Check sheet for the modelled part. Datum: model origin and axes. Units: mm. Face numbers are marked on the shaded views. A direction names the side the tool comes from. Round coordinates to 2 decimals unless told otherwise and drop trailing zeros. Order: outer loops, then holes, each group sorted by start corner. A loop starts at its lowest first (then second) coordinate and runs counter-clockwise, first axis right, second up. Notation, with made-up numbers: (36.25, -3.75) -> (41.25, -3.75) arc R24 ccw to (41.25, 24.25) -> close; hole circle Ø2 at (39, 85.5). An arc over 180 degrees is marked (long way). Use CSV: the item, a comma, the result in double quotes.
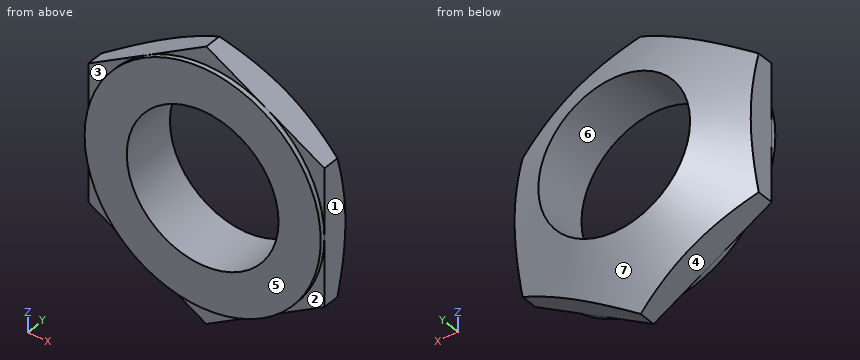
Autodesk Inventor part; units mm, degrees
ref_plane "Work Plane1" through (0, 0, -5.7266) normal (1, 0, 0) x (0, 0, -1)
ref_plane "YZ Plane" through (0, 0, 0) normal (1, 0, 0) x (0, 1, 0)
ref_plane "XZ Plane" through (0, 0, 0) normal (0, 1, 0) x (-1, 0, 0)
sketch "Sketch1" plane through (0, 0, 0) normal (0, 1, 0) x (-1, 0, 0)
  circle A0 centre (0, 0) radius 9.9187
  line L0 (9.9187, -5.7266) -> (0, -11.4531)
  line L1 (0, -11.4531) -> (-9.9187, -5.7266)
  line L2 (-9.9187, -5.7266) -> (-9.9187, 5.7266)
  line L3 (-9.9187, 5.7266) -> (0, 11.4531)
  line L4 (0, 11.4531) -> (9.9187, 5.7266)
  line L5 (9.9187, 5.7266) -> (9.9187, -5.7266)
  line L6 (0, 13.376) -> (0, -12.9473) construction
  point P0 (9.9187, 0)
  dimension "d0" = 19.8374
extrude "Extrusion1" add sketch "Sketch1" along normal blind 4.3688
sketch "Sketch2" plane through (0, 0, 0) normal (0, -1, 0) x (1, 0, 0)
  circle A0 centre (0, 0) radius 9.9187
  line L0 (0, 11.4531) -> (9.9187, 5.7266)
extrude "Extrusion2" add sketch "Sketch2" along normal blind 0.4064
sketch "Sketch3" plane through (0, 4.3688, 0) normal (0, 1, 0) x (1, 0, 0)
  point P0 (0, 0)
  point P1 (0, 0)
hole "Hole1" at (0, 4.3688, 0) direction (0, -1, 0) diameter 12.7508 end through all
thread "Thread1"
ref_plane "Work Plane1" through (0, 0, -5.7266) normal (1, 0, 0) x (0, 0, -1)
sketch "Sketch5" plane through (0, 0, -5.7266) normal (1, 0, 0) x (0, 0, -1)
  line L0 (-12.102, 4.3688) -> (0.6488, 4.3688)
  line L1 (-12.102, 4.3688) -> (-17.1797, 4.3688)
  line L2 (-12.102, 4.3688) -> (-17.1797, 1.4372)
  line L3 (-17.1797, 1.4372) -> (-17.1797, 4.3688)
  line L4 (-5.7266, 0) -> (-5.7266, 18.228)
  dimension "d17" = 30
revolve "Revolution1" cut sketch "Sketch5" angle 360 about axis through (0, 0, 0) along (0, 1, 0)
properties part number "13_8"
Q1. Go/stop test with flat-tipped pins: pin 1 (1 mm diameter, centred on x = -7, y = 1.5, fed in from +Z); pin 2 (0.9 mm diameter, centred on x = 1.5, z = -10.5, fed in from -Y); pin 3 (1 mm diameter, centred on y = 2.5, z = -7, fed in from +X). Record where each tip stops, or that it passes through.
Result sheet:
pin 1,"stops at z = 7.7"
pin 2,"stops at y = 0"
pin 3,"stops at x = 7.88"
Q2. Scan lines: L1, parallel to X at y = 2.25, z = 0; L2, parallel to X at y = 2.65, z = 1.5; L3, parallel to Z at x = -1.25, y = 3.1. Record each from-to range of solid material in increasing order.
Result sheet:
L1,"x = -9.92 to -6.38, 6.38 to 9.92"
L2,"x = -9.23 to -6.2, 6.2 to 9.23"
L3,"z = -8.48 to -6.25, 6.25 to 8.48"
Q3. Access from +Z, -Z, +X, -X, +Y, -Y to the whole of each face (thin tool, end or side, straight path). Record for the marked faces 1, 2 and 3.
Result sheet:
face 1,"+Z, -Z, +X, +Y, -Y"
face 2,"-Z, +X, -Y"
face 3,"+Z, -X, -Y"
Q4. Sectioned sample at B-B, the plane y = 3.5. Enter the section's corners in (x, z).
Result sheet:
outline,"circle Ø15.76 at (0, 0); hole circle Ø12.75 at (0, 0)"
Q5. Sectioned sample at A-A, the plane y = 0.5. Enter the section's corners in (x, z).
Result sheet:
outline,"(-9.92, -5.73) -> (0, -11.45) -> (9.92, -5.73) -> (9.92, 5.73) -> (0, 11.45) -> (-9.92, 5.73) -> close; hole circle Ø12.75 at (0, 0)"
Q6. Mould release check, pull along Z, two halves, no side actions. Record for the marked faces 4, 5, 6 and 7: pulls with the +Z half, pulls with the -Z half, needs draft (parallel to the pull), parting line crosses it, or undercut.
Result sheet:
face 4,"pulls with the -Z half"
face 5,"needs draft"
face 6,"undercut"
face 7,"parting line crosses it"
